The listing builds one solid part. Answer for the finished solid, in the listing's coordinates (mm). A direction names the side the tool comes from. Round coordinates to 2 decimals unless told otherwise and drop trailing zeros. Order: outer loops, then holes, each group sorted by start corner. A loop starts at its lowest first (then second) coordinate and runs counter-clockwise, first axis right, second up. Notation, with made-up numbers: M -5.5,78.25 L 35.5,78.25 A25 ccw 35.5,112.25 Z; hole C 48,-26.75 d8. An arc over 180 degrees is marked long. Write item = value, one per line. Start each with the question number.
(1) Straight lines are drawn through the part: probe 1 along X at (y, z) = (11, -80); probe 2 along Y at (x, z) = (78, 75.5); probe 3 along Z at (x, y) = (82, 13). For each, find the intervals that lie inside material, in ascending order. Write a range as from..to.
(2) For a pull along X with two mould halves and no side action, classify faces 1 (the face through (-79.9, 10.1, 77.5)), 2 (the face through (1, 10, -100)), 3 (the face through (96.99, 9.86, 97.15)), 4 (the face through (-100, 10, -1)) as released by +X, released by -X, zero draft, split by the parting line, or undercut.
(3) A cutting plane is placed at D-D, the plane z = 0. Determine the outline of the cut face in (x, y).
(4) Each of these flat-tipped pins is pushed along its axis until it touches: pin 1 (6.5 mm diameter, centred on x = 80, z = 80, fed in from -Y); pin 2 (10 mm diameter, centred on y = 39.5, z = 1.5, fed in from -X); pin 3 (10 mm diameter, centred on y = 42.5, z = -14.5, fed in from -X); pin 4 (4 mm diameter, centred on x = -80, z = -80, fed in from -Y). Where does it stop, or does it pass through?
(5) A cutting plane is placed at C-C, the plane x = 0. Determine the outline of the cut face in (y, z).
(6) Which of the six approach directions +Z, -Z, +X, -X, +Y, -Y give full straight-line access (tool end or side, diameter ignored) to faces 5 (the face through (97.15, 9.86, -96.99)), 6 (the face through (-1, 20, -46))?
(7) A cutting plane is placed at A-A, the plane z = 80. Determine the outline of the cut face in (x, y).
(8) A cutting plane is placed at B-B, the plane x = 80. Determine the outline of the cut face in (y, z), and give its area (3 significant figures).
from build123d import *

# Parameters (mm, degrees)
BOSS_EXTRUDE1_DEPTH = 20
SKETCH2_R           = 37.5
BOSS_EXTRUDE2_DEPTH = 40
CUT_EXTRUDE1_REACH  = 148.969
SKETCH3_R           = 2.5


with BuildPart() as part:
    # Sketch1 → Boss-Extrude1 (new body)
    with BuildSketch(Plane(origin=(0, 0, 0), x_dir=(1, 0, 0), z_dir=(0, 1, 0))):
        with BuildLine():
            Line((-90, -100), (90, -100))
            ThreePointArc((90, -100), (97.071067812, -97.071067812), (100, -90))
            Line((100, -90), (100, 90))
            ThreePointArc((100, 90), (97.071067812, 97.071067812), (90, 100))
            Line((90, 100), (-90, 100))
            ThreePointArc((-90, 100), (-97.071067812, 97.071067812), (-100, 90))
            Line((-100, 90), (-100, -90))
            ThreePointArc((-100, -90), (-97.071067812, -97.071067812), (-90, -100))
        make_face()
    extrude(amount=BOSS_EXTRUDE1_DEPTH)

    # Sketch2 → Boss-Extrude2 (add)
    with BuildSketch(Plane(origin=(0, 20, 0), x_dir=(1, 0, 0), z_dir=(0, 1, 0))):
        with Locations(Location((0, 0, 0), (0, 0, 270))):
            Circle(SKETCH2_R)
    extrude(amount=BOSS_EXTRUDE2_DEPTH)

    # Sketch3 → Cut-Extrude1 (cut, up to next)
    with BuildSketch(Plane(origin=(0, 20, 0), x_dir=(1, 0, 0), z_dir=(0, 1, 0)), mode=Mode.PRIVATE) as cut_extrude1_sk1:
        with Locations(Location((-80, 80, 0), (0, 0, 270))):
            Circle(SKETCH3_R)
    cut_extrude1_tool1 = extrude(cut_extrude1_sk1.sketch, amount=-CUT_EXTRUDE1_REACH, mode=Mode.PRIVATE) & part.part
    # Sketch3 → Cut-Extrude1 (cut, up to next)
    with BuildSketch(Plane(origin=(0, 20, 0), x_dir=(1, 0, 0), z_dir=(0, 1, 0)), mode=Mode.PRIVATE) as cut_extrude1_sk2:
        with Locations(Location((80, 80, 0), (0, 0, 270))):
            Circle(SKETCH3_R)
    cut_extrude1_tool2 = extrude(cut_extrude1_sk2.sketch, amount=-CUT_EXTRUDE1_REACH, mode=Mode.PRIVATE) & part.part
    # Sketch3 → Cut-Extrude1 (cut, up to next)
    with BuildSketch(Plane(origin=(0, 20, 0), x_dir=(1, 0, 0), z_dir=(0, 1, 0)), mode=Mode.PRIVATE) as cut_extrude1_sk3:
        with Locations(Location((80, -80, 0), (0, 0, 270))):
            Circle(SKETCH3_R)
    cut_extrude1_tool3 = extrude(cut_extrude1_sk3.sketch, amount=-CUT_EXTRUDE1_REACH, mode=Mode.PRIVATE) & part.part
    # Sketch3 → Cut-Extrude1 (cut, up to next)
    with BuildSketch(Plane(origin=(0, 20, 0), x_dir=(1, 0, 0), z_dir=(0, 1, 0)), mode=Mode.PRIVATE) as cut_extrude1_sk4:
        with Locations(Location((-80, -80, 0), (0, 0, 270))):
            Circle(SKETCH3_R)
    cut_extrude1_tool4 = extrude(cut_extrude1_sk4.sketch, amount=-CUT_EXTRUDE1_REACH, mode=Mode.PRIVATE) & part.part
    add(cut_extrude1_tool1.solids().sort_by_distance((-80, 20, -80))[0], mode=Mode.SUBTRACT)
    add(cut_extrude1_tool2.solids().sort_by_distance((80, 20, -80))[0], mode=Mode.SUBTRACT)
    add(cut_extrude1_tool3.solids().sort_by_distance((80, 20, 80))[0], mode=Mode.SUBTRACT)
    add(cut_extrude1_tool4.solids().sort_by_distance((-80, 20, 80))[0], mode=Mode.SUBTRACT)


solid = part.part
Reported:
q1.probe_1 = -100..-82.5, -77.5..77.5, 82.5..100
q1.probe_2 = 0..20
q1.probe_3 = -100..-81.5, -78.5..78.5, 81.5..100
q2.face_1 = undercut
q2.face_2 = zero draft
q2.face_3 = released by +X
q2.face_4 = released by -X
q3.outline = M -100,0 L 100,0 L 100,20 L 37.5,20 L 37.5,60 L -37.5,60 L -37.5,20 L -100,20 Z
q4.pin_1 = 0
q4.pin_2 = -37.5
q4.pin_3 = -36.28
q4.pin_4 = through
q5.outline = M 0,-100 L 20,-100 L 20,-37.5 L 60,-37.5 L 60,37.5 L 20,37.5 L 20,100 L 0,100 Z
q6.face_5 = -Z, +X, +Y, -Y
q6.face_6 = +Y
q7.outline = M -100,0 L -82.5,0 L -82.5,20 L -100,20 Z; M -77.5,0 L 77.5,0 L 77.5,20 L -77.5,20 Z; M 82.5,0 L 100,0 L 100,20 L 82.5,20 Z
q8.outline = M 0,-100 L 20,-100 L 20,-82.5 L 0,-82.5 Z; M 0,-77.5 L 20,-77.5 L 20,77.5 L 0,77.5 Z; M 0,82.5 L 20,82.5 L 20,100 L 0,100 Z
q8.area = 3,800 mm²
